Geometry: final body of the model. Coordinates: model frame, mm. Give positions to 0.01 mm unless a question says otherwise; leave off trailing zeros. Write each loop counter-clockwise with the first axis right and the second up, starting at its lowest first coordinate (ties: lowest second). Pieces come first, ordered by that corner, then holes. Notation, with made-up numbers: (63.5, 46.5) - (95.5, 46.5) arc R7 cw to (95.5, 54.5) - close; hole circle Ø6 at (-6.75, 37.5). An arc over 180 degrees is marked (long way). Return JSON: item names as keys, results as strings.
from build123d import *

# Parameters (mm, degrees)
BOSS_EXTRUDE1_DEPTH = 2.6


with BuildPart() as part:
    # Model → Boss-Extrude1 (new body)
    with BuildSketch(Plane.XY):
        with BuildLine():
            Line((93.65, 50.766666667), (93.65, 122.3))
            Line((93.65, 122.3), (98.51, 122.3))
            ThreePointArc((98.51, 122.3), (99.924213562, 122.885786438), (100.51, 124.3))
            Line((100.51, 124.3), (100.51, 135.3))
            ThreePointArc((100.51, 135.3), (99.924213562, 136.714213562), (98.51, 137.3))
            Line((98.51, 137.3), (93.65, 137.3))
            Line((93.65, 137.3), (93.65, 150))
            Line((93.65, 150), (-93.65, 150))
            Line((-93.65, 150), (-93.65, 137.3))
            Line((-93.65, 137.3), (-98.51, 137.3))
            ThreePointArc((-98.51, 137.3), (-99.924213562, 136.714213562), (-100.51, 135.3))
            Line((-100.51, 135.3), (-100.51, 124.3))
            ThreePointArc((-100.51, 124.3), (-99.924213562, 122.885786438), (-98.51, 122.3))
            Line((-98.51, 122.3), (-93.65, 122.3))
            Line((-93.65, 122.3), (-93.65, 50.766666667))
            Line((-93.65, 50.766666667), (-98.51, 50.766666667))
            ThreePointArc((-98.51, 50.766666667), (-99.924213562, 50.180880229), (-100.51, 48.766666667))
            Line((-100.51, 48.766666667), (-100.51, 37.766666667))
            ThreePointArc((-100.51, 37.766666667), (-99.924213562, 36.352453104), (-98.51, 35.766666667))
            Line((-98.51, 35.766666667), (-93.65, 35.766666667))
            Line((-93.65, 35.766666667), (-93.65, -35.766666667))
            Line((-93.65, -35.766666667), (-98.51, -35.766666667))
            ThreePointArc((-98.51, -35.766666667), (-99.924213562, -36.352453104), (-100.51, -37.766666667))
            Line((-100.51, -37.766666667), (-100.51, -48.766666667))
            ThreePointArc((-100.51, -48.766666667), (-99.924213562, -50.180880229), (-98.51, -50.766666667))
            Line((-98.51, -50.766666667), (-93.65, -50.766666667))
            Line((-93.65, -50.766666667), (-93.65, -122.3))
            Line((-93.65, -122.3), (-98.51, -122.3))
            ThreePointArc((-98.51, -122.3), (-99.924213562, -122.885786438), (-100.51, -124.3))
            Line((-100.51, -124.3), (-100.51, -135.3))
            ThreePointArc((-100.51, -135.3), (-99.924213562, -136.714213562), (-98.51, -137.3))
            Line((-98.51, -137.3), (-93.65, -137.3))
            Line((-93.65, -137.3), (-93.65, -150))
            Line((-93.65, -150), (93.65, -150))
            Line((93.65, -150), (93.65, -137.3))
            Line((93.65, -137.3), (98.51, -137.3))
            ThreePointArc((98.51, -137.3), (99.924213562, -136.714213562), (100.51, -135.3))
            Line((100.51, -135.3), (100.51, -124.3))
            ThreePointArc((100.51, -124.3), (99.924213562, -122.885786438), (98.51, -122.3))
            Line((98.51, -122.3), (93.65, -122.3))
            Line((93.65, -122.3), (93.65, -50.766666667))
            Line((93.65, -50.766666667), (98.51, -50.766666667))
            ThreePointArc((98.51, -50.766666667), (99.924213562, -50.180880229), (100.51, -48.766666667))
            Line((100.51, -48.766666667), (100.51, -37.766666667))
            ThreePointArc((100.51, -37.766666667), (99.924213562, -36.352453104), (98.51, -35.766666667))
            Line((98.51, -35.766666667), (93.65, -35.766666667))
            Line((93.65, -35.766666667), (93.65, 35.766666667))
            Line((93.65, 35.766666667), (98.51, 35.766666667))
            ThreePointArc((98.51, 35.766666667), (99.924213562, 36.352453104), (100.51, 37.766666667))
            Line((100.51, 37.766666667), (100.51, 48.766666667))
            ThreePointArc((100.51, 48.766666667), (99.924213562, 50.180880229), (98.51, 50.766666667))
            Line((98.51, 50.766666667), (93.65, 50.766666667))
        make_face()
    extrude(amount=BOSS_EXTRUDE1_DEPTH)


solid = part.part
Q1. Material intervals for probe 1 along X at (y, z) = (108.5, 0.2), sorted ascending. Write a range as [from, to].
Answer key:
{"probe 1": "x = [-93.65, 93.65]"}
Q2. Section query A-A, the plane y = -97. Return the cut outline in (x, z).
Answer key:
{"outline": "(-93.65, 0) - (93.65, 0) - (93.65, 2.6) - (-93.65, 2.6) - close"}
Q3. Pin query (flat end, axial travel): P1, Ø1, axis at y = -71, z = 2, coming from the -X side; P2, Ø0.8, axis at y = 144, z = 1, coming from the +X side; P3, Ø1.3, axis at x = 96.5, z = 1, coming from the +Y side. Return the tip coordinate at first contact, or that it passes through.
Answer key:
{"P1": "stops at x = -93.65", "P2": "stops at x = 93.65", "P3": "stops at y = 137.3"}
